Autodesk Fusion 360 part; units mm, degrees
sketch "Sketch1" plane through (0, 0, 0) normal (0, 0, 1) x (1, 0, 0)
  circle A0 centre (0, 0) radius 2.25
  circle A1 centre (0, 0) radius 3.15
  circle A2 centre (0, 0) radius 4.55
  circle A3 centre (0, 0) radius 1.15
  dimension "d1" = 9.1
  dimension "d2" = 6.3
  dimension "d3" = 4.5
  dimension "d4" = 2.3
extrude "Extrude1" add sketch "Sketch1" along normal blind 4.3 contours A0 | A1 | A2 | A3
extrude "Extrude2" add sketch "Sketch1" along normal blind 14.9 contours A0 | A1 | A3
extrude "Extrude3" add sketch "Sketch1" along normal blind 21.6 contours A0 | A3
extrude "Extrude4" cut sketch "Sketch1" along normal up to surface (17.3 mm away) from surface at 4.3 contours A3
chamfer "Chamfer1" distance 1 distance2 2.5 1 edges at (-2.0977, -0.8136, 21.6) measured on face at (1.875, -0.1118, 21.6)
Design review of the part built by this model. Coordinates are the model's own, in mm. Round coordinates to 2 decimals unless told otherwise and drop trailing zeros. Write each loop counter-clockwise with the first axis right and the second up, starting at its lowest first coordinate (ties: lowest second). Pieces come first, ordered by that corner, then holes.
Item 1: Consider section C-C on z = 8.5. Give the boundary of the cut face in (x, y).
Item 2: For pin 1 Ø1.8 at (x, y) = (0, 0) entering from +Z; pin 2 Ø2 at (y, z) = (1, 10) entering from -X, all flat-tipped, find the tip position at first contact; note any pin that passes through.
Item 3: Consider section A-A on x = 0. Give the boundary of the cut face in (y, z).
Item 4: Consider section D-D on z = 3.5. Give the boundary of the cut face in (x, y), and give its area (3 significant figures).
Item 5: Draft analysis for pull direction Y (two halves, no side actions). For faces 1 (the cylindrical face through (-0.99, 4.44, 2.12)), 2 (the cylindrical face through (-0.91, 0.7, 12.83)), 3 (the flat face through (0, 0, 0)), state which applies: released by +Y, released by -Y, zero draft, split by the parting line, or undercut.
Item 6: Wall thickness on L1, parallel to Y at x = 0, z = 13.5; L2, parallel to Y at x = 0, z = 15; L3, parallel to Z at x = 4, y = 0: over which ranges is each line inside the solid? List them lowest first.
Check values:
1. outline: circle Ø6.3 at (0, 0); hole circle Ø2.3 at (0, 0)
2. pin 1: stops at z = 4.3
2. pin 2: stops at x = -3.15
3. outline: (-4.55, 0) - (4.55, 0) - (4.55, 4.3) - (3.15, 4.3) - (3.15, 14.9) - (2.25, 14.9) - (2.25, 19.1) - (1.25, 21.6) - (1.15, 21.6) - (1.15, 4.3) - (-1.15, 4.3) - (-1.15, 21.6) - (-1.25, 21.6) - (-2.25, 19.1) - (-2.25, 14.9) - (-3.15, 14.9) - (-3.15, 4.3) - (-4.55, 4.3) - close
4. outline: circle Ø9.1 at (0, 0)
4. area: 65.0 mm2
5. face 1: split by the parting line
5. face 2: undercut
5. face 3: zero draft
6. L1: y = -3.15 to -1.15, 1.15 to 3.15
6. L2: y = -2.25 to -1.15, 1.15 to 2.25
6. L3: z = 0 to 4.3
